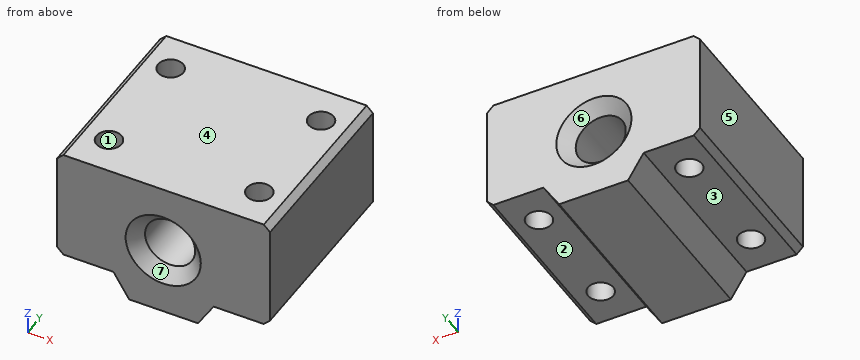
```python
from build123d import *

# Parameters (mm, degrees)
F0_R     = 4
F1_DEPTH = 30
F2_SIZE  = 2
F3_SIZE  = 1
F4_R     = 2
F5_DEPTH = 25


with BuildPart() as f1:
    # F0 (on Front) → F1 (new body)
    with BuildSketch(Plane.XZ):
        Polygon((-12.461195, 38.328968), (-46.461195, 38.328968), (-46.461195, 20.328968), (-37.461195, 20.328968), (-34.961195, 16.328968), (-23.961195, 16.328968), (-21.461195, 20.328968), (-12.461195, 20.328968), align=None)
        with Locations((-29.514153, 27.328968)):
            Circle(F0_R, mode=Mode.SUBTRACT)
    extrude(amount=F1_DEPTH)

    # F2
    f2_edges = [f1.edges().sort_by_distance(p)[0] for p in [
        (-33.514153, -30, 27.328968),
        (-33.514153, 0, 27.328968),
    ]]
    chamfer(f2_edges, length=F2_SIZE)

    # F3
    f3_edges = [f1.edges().sort_by_distance(p)[0] for p in [
        (-46.461195, -15, 38.328968),
        (-12.461195, -15, 38.328968),
        (-12.461195, -15, 20.328968),
        (-46.461195, -15, 20.328968),
    ]]
    chamfer(f3_edges, length=F3_SIZE)

    # F4 (on face) → F5 (cut)
    with BuildSketch(Plane.XY.offset(38.328968)):
        with Locations((-41.461195, -6)):
            Circle(F4_R)
        with Locations((-41.461195, -24)):
            Circle(F4_R)
        with Locations((-17.461195, -24)):
            Circle(F4_R)
        with Locations((-17.461195, -6)):
            Circle(F4_R)
    extrude(amount=-F5_DEPTH, mode=Mode.SUBTRACT)


solid = f1.part
```
Source: CAD feature listing. Evaluate the final solid. Frame: model axes, mm. Face numbers are marked on the shaded views. A direction names the side the tool comes from. Give positions to 0.01 mm unless a question says otherwise; leave off trailing zeros. Write each loop counter-clockwise with the first axis right and the second up, starting at its lowest first coordinate (ties: lowest second). Pieces come first, ordered by that corner, then holes. Notation, with made-up numbers: (79.25, 30) - (95.25, 30) arc R26 ccw to (95.25, 53) - close; hole circle Ø2 at (84.5, 76.25). An arc over 180 degrees is marked (long way). One line per item, written item: value. Start each with the question number.
Q1. Section query D-D, the plane x = -20. Return the cut outline in (y, z), then the cut area to 3 significant figures.
Q2. Section query C-C, the plane y = -24.5. Return the cut outline in (x, z), then the cut area to 3 significant figures.
Q3. Draft query along Z for the marked faces 4, 5, 6 and 7. Return one class per face: +Z half, -Z half, draft (parallel to the pull), parting line (faces both ways), or undercut.
Q4. Section query B-B, the plane z = 34.25. Return the cut outline in (x, y), then the cut area to 3 significant figures.
Q5. Set-up query: the marked faces 1, 2 and 3. Return all of +Z, -Z, +X, -X, +Y, -Y with unobstructed straight access to the full face (end or side cutting, diameter ignored); none if empty.
Q6. First-contact query: pin 1 Ø2.5 at (x, y) = (-17, -16.5) entering from -Z; pin 2 Ø3.5 at (x, y) = (-17.46, -24) entering from -Z. Flat tips, straight axial feed; report the tip coordinate or a pass-through.
Q7. Section query A-A, the plane y = -6. Return the cut outline in (x, z).
Q8. Material intervals for probe 1 along Y at (x, z) = (-17.5, 30.25); probe 2 along Y at (x, z) = (-40, 32); probe 3 along X at (y, z) = (-25.25, 20.75), sorted ascending. Write a range as from..to.
Answer:
1. outline: (-30, 20.33) - (0, 20.33) - (0, 38.33) - (-30, 38.33) - close
1. area: 540 mm2
2. outline: (-46.46, 21.33) - (-45.46, 20.33) - (-43.4, 20.33) - (-43.4, 38.33) - (-45.46, 38.33) - (-46.46, 37.33) - close; (-39.52, 20.33) - (-37.46, 20.33) - (-34.96, 16.33) - (-23.96, 16.33) - (-21.46, 20.33) - (-19.4, 20.33) - (-19.4, 38.33) - (-39.52, 38.33) - close; (-15.52, 20.33) - (-13.46, 20.33) - (-12.46, 21.33) - (-12.46, 37.33) - (-13.46, 38.33) - (-15.52, 38.33) - close; hole circle Ø8 at (-29.51, 27.33)
2. area: 474 mm2
3. face 4: +Z half
3. face 5: draft
3. face 6: undercut
3. face 7: undercut
4. outline: (-46.46, -30) - (-12.46, -30) - (-12.46, 0) - (-46.46, 0) - close; hole circle Ø4 at (-41.46, -24); hole circle Ø4 at (-41.46, -6); hole circle Ø4 at (-17.46, -24); hole circle Ø4 at (-17.46, -6)
4. area: 970 mm2
5. face 1: +Z, -Z
5. face 2: -Z, +X, +Y, -Y
5. face 3: -Z, -X, +Y, -Y
6. pin 1: stops at z = 20.33
6. pin 2: passes through
7. outline: (-46.46, 21.33) - (-45.46, 20.33) - (-43.46, 20.33) - (-43.46, 38.33) - (-45.46, 38.33) - (-46.46, 37.33) - close; (-39.46, 20.33) - (-37.46, 20.33) - (-34.96, 16.33) - (-23.96, 16.33) - (-21.46, 20.33) - (-19.46, 20.33) - (-19.46, 38.33) - (-39.46, 38.33) - close; (-15.46, 20.33) - (-13.46, 20.33) - (-12.46, 21.33) - (-12.46, 37.33) - (-13.46, 38.33) - (-15.46, 38.33) - close; hole circle Ø8 at (-29.51, 27.33)
8. probe 1: y = -30..-26, -22..-8, -4..0
8. probe 2: y = -30..-25.37, -22.63..-7.37, -4.63..0
8. probe 3: x = -45.88..-43.02, -39.9..-19.02, -15.9..-13.04
